Autodesk Inventor part; units mm, degrees
ref_plane "YZ Plane" through (0, 0, 0) normal (1, 0, 0) x (0, 1, 0)
ref_plane "XZ Plane" through (0, 0, 0) normal (0, 1, 0) x (-1, 0, 0)
ref_plane "XY Plane" through (0, 0, 0) normal (0, 0, 1) x (1, 0, 0)
sketch "Sketch1" plane through (0, 0, 0) normal (1, 0, 0) x (0, 1, 0)
  line L0 (0, 0) -> (77, 0)
  line L1 (77, 0) -> (77, -23)
  line L2 (77, -23) -> (0, -23)
  line L3 (0, -23) -> (0, 0)
  line L4 (71, -11.5) -> (71, -8)
  line L5 (71, -8) -> (71, -15)
  line L6 (71, -15) -> (77, -15)
  line L7 (71, -8) -> (77, -8)
  line L8 (0, -8) -> (6, -8)
  line L9 (6, -8) -> (6, -15)
  line L10 (6, -15) -> (0, -15)
  circle A0 centre (59, -11.5) radius 5
  dimension "d0" = 77
  dimension "d1" = 23
  dimension "d3" = 3.5
  dimension "d4" = 7
  dimension "d5" = 6
  dimension "d6" = 7
  dimension "d10" = 10
extrude "Extrusion1" add sketch "Sketch1" along normal blind 6 contours L0 L1 L7 L4 L5 L6 L2 L3 L10 L9 L8 | A0
sketch "Sketch2" plane through (6, 0, 0) normal (1, 0, 0) x (0, 0, -1)
  line L0 (15, 71) -> (8, 71)
  circle A0 centre (11.5, 59) radius 5
  point P0 (0, 0)
  dimension "d12" = 10
extrude "Extrusion2" cut sketch "Sketch2" against normal blind 6
sketch "Sketch3" plane through (6, 0, 0) normal (1, 0, 0) x (0, 0, -1)
  line L0 (8, 6) -> (15, 6)
  line L1 (11.5, 16) -> (6.5, 16)
  line L2 (6.5, 16) -> (6.5, 22)
  line L3 (6.5, 22) -> (16.5, 22)
  line L4 (16.5, 22) -> (16.5, 16)
  line L5 (16.5, 16) -> (11.5, 16)
  line L6 (11.5, 37) -> (16.5, 37)
  line L7 (16.5, 37) -> (16.5, 43)
  line L8 (16.5, 43) -> (6.5, 43)
  line L9 (6.5, 43) -> (6.5, 37)
  line L10 (6.5, 37) -> (11.5, 37)
  point P0 (0, 0)
  dimension "d16" = 5
  dimension "d17" = 6
  dimension "d18" = 10
  dimension "d19" = 6
  dimension "d21" = 5
  dimension "d22" = 6
  dimension "d23" = 10
  dimension "d24" = 6
extrude "Extrusion3" cut sketch "Sketch3" against normal blind 6
properties part number "g_arm3"
Work out the finished part from the listing and answer in its coordinate system (mm). A direction names the side the tool comes from. Give positions to 0.01 mm unless a question says otherwise; leave off trailing zeros. Loops run counter-clockwise (first coordinate to the right, second up) from the corner with the lowest first, then second, coordinate; pieces in that order, holes last. Notation, with made-up numbers: (17.5, 49.5) - (67.5, 49.5) arc R18 cw to (67.5, 69.5) - close; hole circle Ø5 at (61.25, 69.5). An arc over 180 degrees is marked (long way). Answer in a Markdown table with one row per item. Add a question column.
Q1. The part is cut by section B-B (z = -11.5). Determine the outline of the cut face in (x, y), and give its area (3 significant figures).
Q2. A tool of negligible diameter and unlimited length cuts with its end or side. For faces 5 (the flat face through (3, 3, -15)), 6 (the flat face through (3, 71, -12)), 7 (the flat face through (3, 22, -11)), from which of +Z, -Z, +X, -X, +Y, -Y can it reach the whole face along a straight path? Write none if from no direction.
Q3. Each of these flat-tipped pins is pushed along its axis until it touches: P1, Ø1.8, axis at x = 3.5, z = -10, coming from the -Y side; P2, Ø1.8, axis at x = 2, z = -11.5, coming from the +Y side. Where does it stop, or does it pass through?
Q4. The part is cut by section A-A (y = 59). Determine the outline of the cut face in (x, z).
Q5. Determine the mould class of faces 1 (the flat face through (3, 74, -8)), 2 (the flat face through (3, 37, -11)), 3 (the flat face through (3, 6, -11)), 4 (the flat face through (3, 16, -12)) for opening direction Y: released by +Y, released by -Y, zero draft, split by the parting line, or undercut.
Q6. Consider line 1 along Y through (x, z) = (4, -11.5); line 2 along Y through (x, z) = (4.8, -14.5). Determine where each line is inside the solid, lowest interval first.
Q7. The part is cut by section D-D (y = 72.5). Determine the outline of the cut face in (x, z), and give its area (3 significant figures).
Q8. The part is cut by section C-C (x = 1.4). Determine the outline of the cut face in (y, z), and give its area (3 significant figures).
Solution:
| question | item | result |
|---|---|---|
| 1 | outline | (0, 6) - (6, 6) - (6, 16) - (0, 16) - close; (0, 22) - (6, 22) - (6, 37) - (0, 37) - close; (0, 43) - (6, 43) - (6, 54) - (0, 54) - close; (0, 64) - (6, 64) - (6, 71) - (0, 71) - close |
| 1 | area | 258 mm² |
| 2 | face 5 | +X, -X, -Y |
| 2 | face 6 | +X, -X, +Y |
| 2 | face 7 | +X, -X |
| 3 | P1 | stops at y = 6 |
| 3 | P2 | stops at y = 71 |
| 4 | outline | (0, -23) - (6, -23) - (6, -16.5) - (0, -16.5) - close; (0, -6.5) - (6, -6.5) - (6, 0) - (0, 0) - close |
| 5 | face 1 | zero draft |
| 5 | face 2 | undercut |
| 5 | face 3 | released by -Y |
| 5 | face 4 | undercut |
| 6 | line 1 | y = 6 to 16, 22 to 37, 43 to 54, 64 to 71 |
| 6 | line 2 | y = 6 to 16, 22 to 37, 43 to 55, 63 to 71 |
| 7 | outline | (0, -23) - (6, -23) - (6, -15) - (0, -15) - close; (0, -8) - (6, -8) - (6, 0) - (0, 0) - close |
| 7 | area | 96.0 mm² |
| 8 | outline | (0, -23) - (77, -23) - (77, -15) - (71, -15) - (71, -8) - (77, -8) - (77, 0) - (0, 0) - (0, -8) - (6, -8) - (6, -15) - (0, -15) - close; hole (16, -16.5) - (22, -16.5) - (22, -6.5) - (16, -6.5) - close; hole (37, -16.5) - (43, -16.5) - (43, -6.5) - (37, -6.5) - close; hole circle Ø10 at (59, -11.5) |
| 8 | area | 1,490 mm² |
